```python
from build123d import *

# Parameters (mm, degrees)
SKETCH1_R           = 2.032
BOSS_EXTRUDE2_DEPTH = 4.064


with BuildPart() as part:
    # Sketch1 → Boss-Extrude2 (new body)
    with BuildSketch(Plane.XY):
        with BuildLine():
            Line((40.64, 5.08), (40.64, 172.72))
            ThreePointArc((40.64, 172.72), (35.432358569, 185.292358569), (22.86, 190.5))
            Line((22.86, 190.5), (17.78, 190.5))
            ThreePointArc((17.78, 190.5), (5.207641431, 185.292358569), (0, 172.72))
            Line((0, 172.72), (0, 5.08))
            ThreePointArc((0, 5.08), (1.487897552, 1.487897552), (5.08, 0))
            Line((5.08, 0), (26.416, 0))
            Line((26.416, 0), (35.56, 0))
            ThreePointArc((35.56, 0), (39.152102448, 1.487897552), (40.64, 5.08))
        make_face()
        with Locations((26.416, 24.13)):
            Circle(SKETCH1_R, mode=Mode.SUBTRACT)
        with Locations((26.416, 64.77)):
            Circle(SKETCH1_R, mode=Mode.SUBTRACT)
        with Locations((26.416, 113.03)):
            Circle(SKETCH1_R, mode=Mode.SUBTRACT)
        with Locations((26.416, 153.67)):
            Circle(SKETCH1_R, mode=Mode.SUBTRACT)
        with Locations((17.272, 3.048)):
            Circle(SKETCH1_R, mode=Mode.SUBTRACT)
        with Locations((13.531045562, 163.449)):
            Circle(SKETCH1_R, mode=Mode.SUBTRACT)
        with Locations((13.492529792, 181.102)):
            Circle(SKETCH1_R, mode=Mode.SUBTRACT)
    extrude(amount=BOSS_EXTRUDE2_DEPTH)


solid = part.part
```
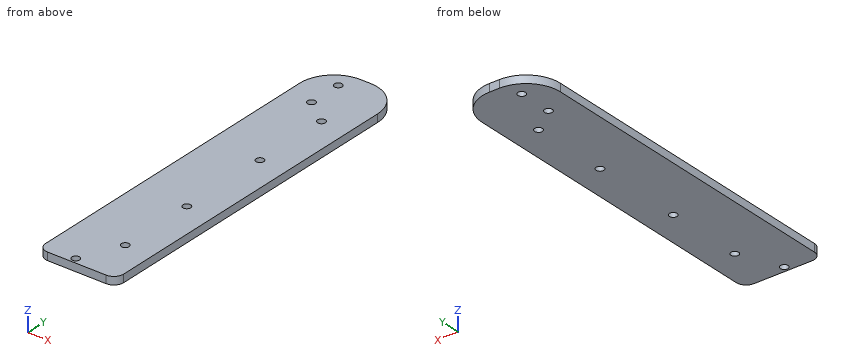
Verification items for the finished model (mm, model axes). Round coordinates to 2 decimals unless told otherwise and drop trailing zeros. Write each loop counter-clockwise with the first axis right and the second up, starting at its lowest first coordinate (ties: lowest second). Pieces come first, ordered by that corner, then holes. Notation, with made-up numbers: (35, -5) - (68, -5) arc R30 cw to (68, 20) - close; hole circle Ø6 at (-2, 35.25). An arc over 180 degrees is marked (long way). Answer as a JSON object with one key per item and string values. Group by question number.
Q1. Section check A-A, the plane y = 64.77. Enter the section's corners in (x, z), plus the area to 3 significant figures.
Q2. Go/stop test with flat-tipped pins: pin 1 Ø2.5 at (x, y) = (13.49, 181.1) entering from -Z; pin 2 Ø6.5 at (x, y) = (26.416, 153.67) entering from -Z. Record where each tip stops, or that it passes through.
Q3. Section check B-B, the plane z = 1.65. Enter the section's corners in (x, y).
Q4. Thickness scan on line 1 (Y direction, x = 25, z = 0.8); line 2 (Y direction, x = 12, z = 3.6); line 3 (Y direction, x = 13.5, z = 2.85). Record the ranges inside material, lowest first.
Found:
{
 "1": {"outline": "(0, 0) - (24.38, 0) - (24.38, 4.06) - (0, 4.06) - close; (28.45, 0) - (40.64, 0) - (40.64, 4.06) - (28.45, 4.06) - close", "area": "149 mm^2"},
 "2": {"pin 1": "passes through", "pin 2": "stops at z = 0"},
 "3": {"outline": "(0, 5.08) arc R5.08 ccw to (5.08, 0) - (35.56, 0) arc R5.08 ccw to (40.64, 5.08) - (40.64, 172.72) arc R17.78 ccw to (22.86, 190.5) - (17.78, 190.5) arc R17.78 ccw to (0, 172.72) - close; hole circle Ø4.06 at (13.49, 181.1); hole circle Ø4.06 at (13.53, 163.45); hole circle Ø4.06 at (17.27, 3.05); hole circle Ø4.06 at (26.42, 24.13); hole circle Ø4.06 at (26.42, 64.77); hole circle Ø4.06 at (26.42, 113.03); hole circle Ø4.06 at (26.42, 153.67)"},
 "4": {"line 1": "y = 0 to 22.67, 25.59 to 63.31, 66.23 to 111.57, 114.49 to 152.21, 155.13 to 190.37", "line 2": "y = 0 to 162.11, 164.79 to 179.72, 182.48 to 189.53", "line 3": "y = 0 to 161.42, 165.48 to 179.07, 183.13 to 189.98"}
}
